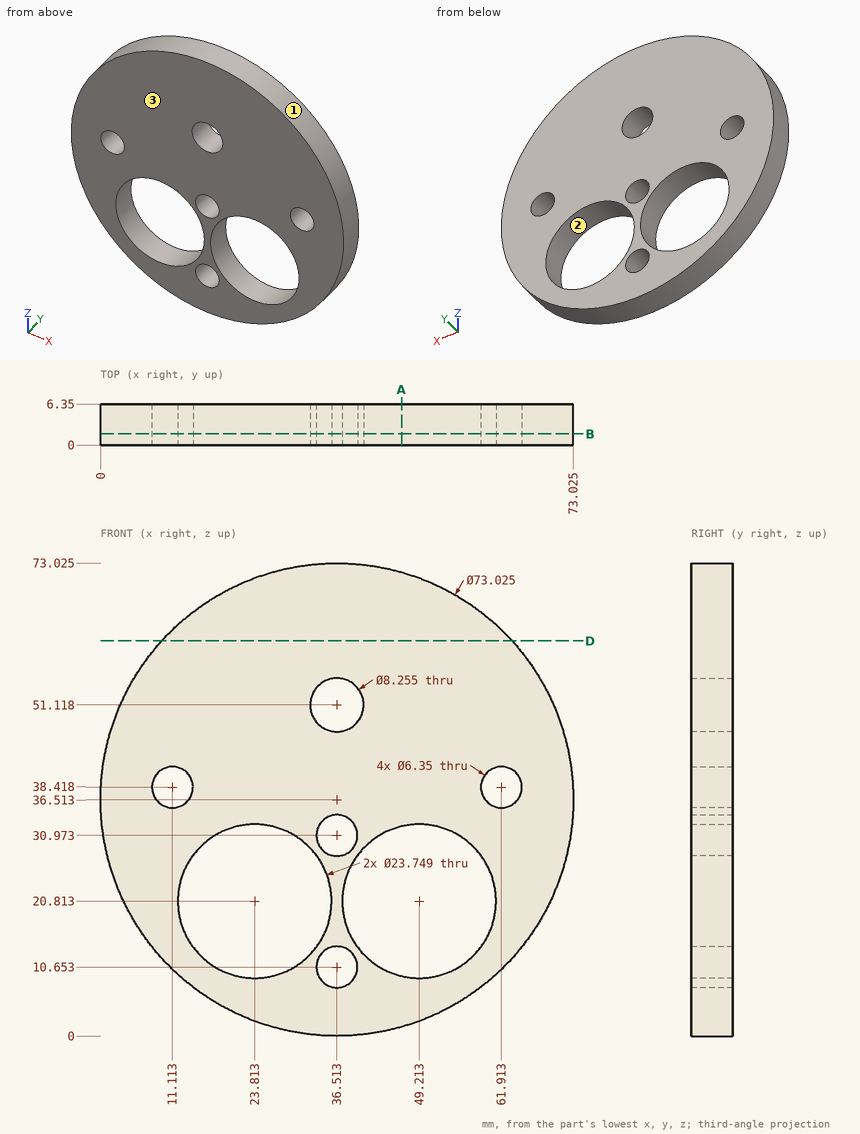
The drawing under review shows one solid part. Ordinate dimensions are in mm from its lowest x, y, z. Round coordinates to 2 decimals unless told otherwise and drop trailing zeros. Write each loop counter-clockwise with the first axis right and the second up, starting at its lowest first coordinate (ties: lowest second). Pieces come first, ordered by that corner, then holes. Notation, with made-up numbers: M -37.5,-17.75 L -24.5,-17.75 A19 cw -24.5,-11.75 Z; hole C 5.25,-40 d3. An arc over 180 degrees is marked long. One line per item, written item: value. Start each with the question number.
(1) We need section B-B (y = 1.75). Count the separate pieces of the cut face and the enclosed holes in it, and give its area (3 significant figures).
(2) Wall thickness on line 1 (X direction, y = 0.5, z = 10.5) (1 decimal); line 2 (X direction, y = 1.5, z = 36.5) (1 decimal); line 3 (X direction, y = 4.25, z = 40) (1 decimal): over which ranges is each line inside the solid? List them lowest first.
(3) We need section D-D (z = 61). Give the boundary of the cut face in (x, y), and give its area (3 significant figures).
(4) We need section A-A (x = 46.5). Give the boundary of the cut face in (y, z), and give its area (3 significant figures).
(5) The part is to be moulded in two halves that separate along X. For the marked faces 1, 2 and 3, say which applies: released by +X, released by -X, zero draft, split by the parting line, or undercut.
(6) Insertion check: pin 1 (2 mm diameter, centred on y = 4, z = 46.5, fed in from -X); pin 2 (8.5 mm diameter, centred on x = 36.51, z = 10.65, fed in from +Y); pin 3 (2 mm diameter, centred on x = 60.5, y = 3, fed in from +Z). Each pin has a flat end and moves straight along its axis. Give the tip position at first contact, or say it passes through.
Result:
1. separate pieces: 1
1. enclosed holes: 7
1. area: 3,120 mm²
2. line 1: 10.9 to 17.9, 29.7 to 33.3, 39.7 to 43.3, 55.1 to 62.1
2. line 2: 0 to 8.6, 13.6 to 59.4, 64.4 to 73
2. line 3: 0.2 to 8.4, 13.9 to 59.2, 64.7 to 72.9
3. outline: M 9.43,0 L 63.6,0 L 63.6,6.35 L 9.43,6.35 Z
3. area: 344 mm²
4. outline: M 0,1.39 L 6.35,1.39 L 6.35,9.25 L 0,9.25 Z; M 0,32.37 L 6.35,32.37 L 6.35,71.63 L 0,71.63 Z
4. area: 299 mm²
5. face 1: split by the parting line
5. face 2: undercut
5. face 3: zero draft
6. pin 1: x = 1.12
6. pin 2: y = 6.35
6. pin 3: z = 64.88
